```python
from build123d import *

# Parameters (mm, degrees)
F2_DEPTH      = 55
F3_DEPTH      = 74.001
F3_DEPTH_BACK = 74.001
F4_DEPTH      = 45


with BuildPart() as f2:
    # F0 (on Front) → F2 (new body, through all)
    with BuildSketch(Plane.XZ):
        Polygon((-72, 137), (-74, 77), (0, 77), (74, 77), (72, 137), (0, 137), align=None)
        Polygon((-74, 77), (-59, 0), (-47, 50), (0, 50), (47, 50), (59, 0), (74, 77), (0, 77), align=None)
    extrude(amount=F2_DEPTH)

    # F1 (on Right) → F3 (cut, two sides)
    with BuildSketch(Plane.YZ) as f3_sk:
        Polygon((-55, 77), (-45, 137), (-80.7239860296, 137), (-80.7239860296, 0), (-33, 0), align=None)
    extrude(amount=-F3_DEPTH, mode=Mode.SUBTRACT)
    extrude(f3_sk.sketch, amount=F3_DEPTH_BACK, mode=Mode.SUBTRACT)

    # F4 (add): a face of the model
    f4_faces = [f2.faces().sort_by_distance(p)[0] for p in [
        (0, 0, 88.8782570615),
    ]]
    extrude(f4_faces, amount=F4_DEPTH)


solid = f2.part
```
The model under review builds one solid part; all positions refer to its coordinate system, in mm. A direction names the side the tool comes from. Give positions to 0.01 mm unless a question says otherwise; leave off trailing zeros. Loops run counter-clockwise (first coordinate to the right, second up) from the corner with the lowest first, then second, coordinate; pieces in that order, holes last. Notation, with made-up numbers: (-9.75, -9.5) -> (45.25, -9.5) arc R25 cw to (45.25, 9.5) -> close; hole circle Ø10 at (-26.75, 51). An arc over 180 degrees is marked (long way). Use CSV: the item, a comma, the result in double quotes.
1. For P1, Ø5, axis at y = 14, z = 109.5, coming from the +X side; P2, Ø10, axis at x = -10.5, y = 3, coming from the -Z side; P3, Ø8, axis at y = -11.5, z = 42, coming from the -X side, all flat-tipped, find the tip position at first contact; note any pin that passes through.
Result:
P1,"stops at x = 73"
P2,"stops at z = 50"
P3,"stops at x = -67.96"
2. To check wall thickness, follow probe 1 along Z at (x, y) = (8, -18); probe 2 along X at (y, z) = (-17, 42); probe 3 along X at (y, z) = (-41, 38.5). State the ranges of each line that lie inside material, in increasing order. Write a range as from..to.
Result:
probe 1,"z = 50..137"
probe 2,"x = -67.18..-48.92, 48.92..67.18"
probe 3,"x = -66.5..-49.76, 49.76..66.5"
3. Machinability: for faces 1 (the face through (1, -1, 137)), 2 (the face through (53, -2, 25)), which of the approach directions +Z, -Z, +X, -X, +Y, -Y give a long, thin tool a straight path to every point of the face, cutting with its end or side? Answer none if there is none.
Result:
face 1,"+Z, +X, -X, +Y, -Y"
face 2,"-Z, +Y, -Y"
4. Consider section C-C, the plane y = -13. Write out the cut boundary in (x, z).
Result:
outline,"(-74, 77) -> (-59, 0) -> (-47, 50) -> (47, 50) -> (59, 0) -> (74, 77) -> (72, 137) -> (-72, 137) -> close"
5. Consider section A-A, the plane z = 13.5. Write out the cut boundary in (x, y).
Result:
outline,"(-61.63, -36.86) -> (-55.76, -36.86) -> (-55.76, 45) -> (-61.63, 45) -> close; (55.76, -36.86) -> (61.63, -36.86) -> (61.63, 45) -> (55.76, 45) -> close"
6. Consider section B-B, the plane x = -33.5. Write out the cut boundary in (y, z).
Result:
outline,"(-55, 77) -> (-47.29, 50) -> (45, 50) -> (45, 137) -> (-45, 137) -> close"
7. Consider section D-D, the plane z = 48. Write out the cut boundary in (x, y).
Result:
outline,"(-68.35, -46.71) -> (-47.48, -46.71) -> (-47.48, 45) -> (-68.35, 45) -> close; (47.48, -46.71) -> (68.35, -46.71) -> (68.35, 45) -> (47.48, 45) -> close"
8. The part is to be moulded in two halves that separate along X. For faces 3 (the face through (-1, -2, 50)), 4 (the face through (66.395, 5.411, 37.961)), 5 (the face through (-1, 45, 85)), 6 (the face through (-53, -2, 25)), say which applies: +X half, -X half, draft (parallel to the pull), parting line (faces both ways), or undercut.
Result:
face 3,"undercut"
face 4,"+X half"
face 5,"draft"
face 6,"undercut"
